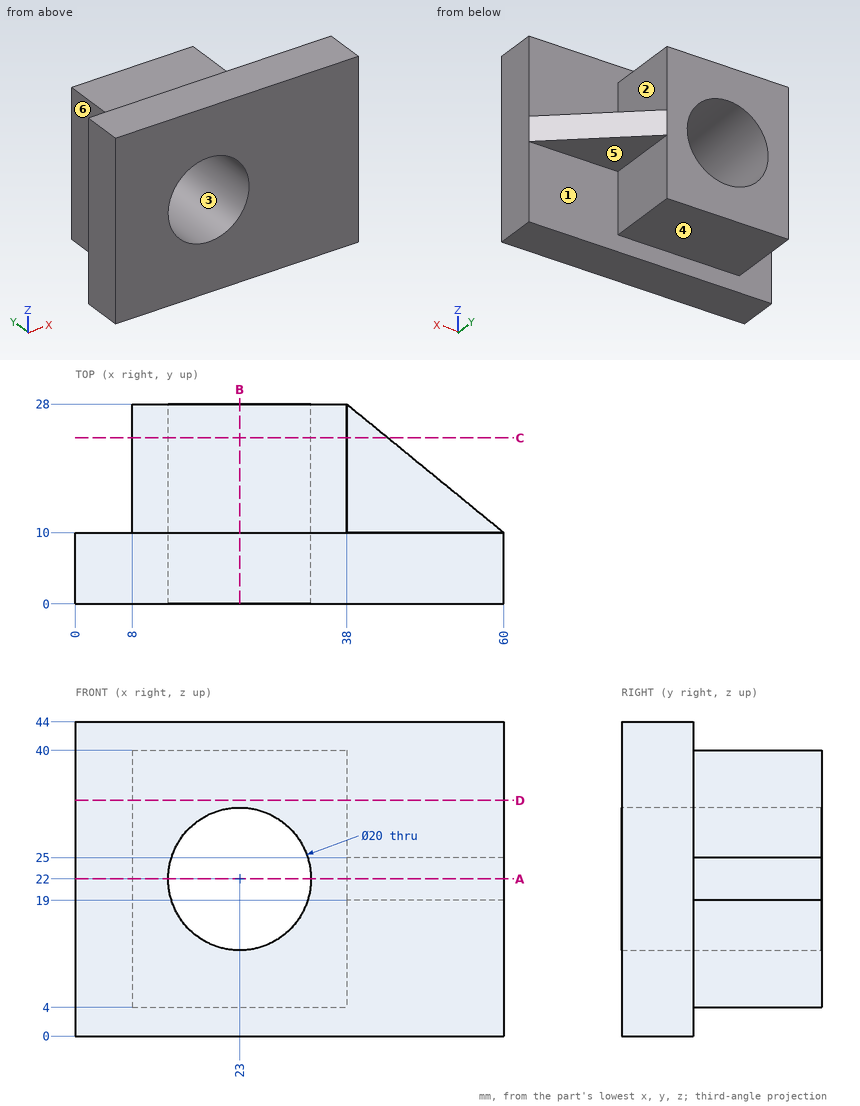
Geometry check sheet. Reference: drawing and pictorial views, mm from the part's lowest x, y, z. A direction names the side the tool comes from. Give positions to 0.01 mm unless a question says otherwise; leave off trailing zeros. Loops run counter-clockwise (first coordinate to the right, second up) from the corner with the lowest first, then second, coordinate; pieces in that order, holes last. Notation, with made-up numbers: (-15, 40.25) -> (42, 40.25) arc R23 ccw to (42, 61.25) -> close; hole circle Ø10 at (69.25, 33.5). An arc over 180 degrees is marked (long way). Answer in a Markdown table with one row per item. Add a question column.
1) Cross-section at C-C on y = 23.25. Record the boundary of the cut face in (x, z), and give its area (3 significant figures).
2) Cross-section at A-A on z = 22. Record the boundary of the cut face in (x, y), and give its area (3 significant figures).
3) Set-up check for the marked faces 4, 5 and 6: record each of +Z, -Z, +X, -X, +Y, -Y from which the full face is reachable in a straight line by a thin tool's end or side.
4) Cross-section at D-D on z = 33. Record the boundary of the cut face in (x, y).
5) Draft check along X on the marked faces 1, 2 and 3. Enter one of: pulls with the +X half, pulls with the -X half, needs draft (parallel to the pull), parting line crosses it, or undercut.
6) Gauge pin test, flat ends, axial feed: P1, Ø5.5, axis at x = 17.5, y = 15.5, coming from the +Z side; P2, Ø1, axis at y = 16, z = 23, coming from the -X side; P3, Ø12, axis at y = 22.5, z = 8, coming from the +X side. Record the tip position at first contact, or that the pin passes through.
7) Material ranges on probe 1 along X at (y, z) = (6.5, 22); probe 2 along Y at (x, z) = (5, 22.5); probe 3 along Z at (x, y) = (31.5, 21.5), recorded low to high. Write a range as from..to.
8) Cross-section at B-B on x = 23. Record the boundary of the cut face in (y, z).
Outcome:
| question | item | result |
|---|---|---|
| 1 | outline | (8, 4) -> (38, 4) -> (38, 19) -> (43.81, 19) -> (43.81, 25) -> (38, 25) -> (38, 40) -> (8, 40) -> close; hole circle Ø20 at (23, 22) |
| 1 | area | 801 mm^2 |
| 2 | outline | (0, 0) -> (13, 0) -> (13, 28) -> (8, 28) -> (8, 10) -> (0, 10) -> close; (33, 0) -> (60, 0) -> (60, 10) -> (38, 28) -> (33, 28) -> close |
| 2 | area | 778 mm^2 |
| 3 | face 4 | -Z, +X, -X, +Y |
| 3 | face 5 | -Z, +X, +Y |
| 3 | face 6 | +Z, -Z, -X, +Y |
| 4 | outline | (0, 0) -> (60, 0) -> (60, 10) -> (38, 10) -> (38, 28) -> (8, 28) -> (8, 10) -> (0, 10) -> close |
| 5 | face 1 | needs draft |
| 5 | face 2 | pulls with the +X half |
| 5 | face 3 | undercut |
| 6 | P1 | stops at z = 40 |
| 6 | P2 | stops at x = 8 |
| 6 | P3 | stops at x = 38 |
| 7 | probe 1 | x = 0..13, 33..60 |
| 7 | probe 2 | y = 0..10 |
| 7 | probe 3 | z = 4..16.73, 27.27..40 |
| 8 | outline | (0, 0) -> (10, 0) -> (10, 4) -> (28, 4) -> (28, 12) -> (0, 12) -> close; (0, 32) -> (28, 32) -> (28, 40) -> (10, 40) -> (10, 44) -> (0, 44) -> close |
